Here's how the part is built. I have some questions about the finished solid (model axes, mm). Round coordinates to 2 decimals unless told otherwise and drop trailing zeros. Write each loop counter-clockwise with the first axis right and the second up, starting at its lowest first coordinate (ties: lowest second). Pieces come first, ordered by that corner, then holes. Notation, with made-up numbers: (35, -32.5) -> (90, -32.5) arc R13 ccw to (90, -28.5) -> close; hole circle Ø3 at (-1, 60.5). An arc over 180 degrees is marked (long way). Answer in a Markdown table with one row per item.
Autodesk Inventor part; units mm, degrees
ref_plane "YZ Plane" through (0, 0, 0) normal (1, 0, 0) x (0, 1, 0)
ref_plane "XZ Plane" through (0, 0, 0) normal (0, 1, 0) x (-1, 0, 0)
ref_plane "XY Plane" through (0, 0, 0) normal (0, 0, 1) x (1, 0, 0)
sketch "スケッチ1" plane through (0, 0, 0) normal (0, 0, 1) x (1, 0, 0)
  line L0 (-145, 50) -> (145, 50)
  line L1 (145, 50) -> (145, -50)
  line L2 (145, -50) -> (-145, -50)
  line L3 (-145, -50) -> (-145, 50)
  line L4 (0, -70) -> (0, 70)
  line L5 (-203, 0) -> (203, 0)
  circle A0 centre (-104.5, 10.5) radius 2.6
  circle A1 centre (-125, 21) radius 5.1
  circle A2 centre (-74.5, 10.5) radius 2.6
  circle A3 centre (-44.5, 10.5) radius 2.6
  circle A4 centre (-14.5, 10.5) radius 2.6
  circle A5 centre (15.5, 10.5) radius 2.6
  circle A6 centre (45.5, 10.5) radius 2.6
  circle A7 centre (75.5, 10.5) radius 2.6
  circle A8 centre (105.5, 10.5) radius 2.6
  line L6 (-25.25, 33.5) -> (25.25, 33.5)
  line L7 (25.25, 33.5) -> (25.25, 30)
  line L8 (25.25, 30) -> (-25.25, 30)
  line L9 (-25.25, 30) -> (-25.25, 33.5)
  circle A9 centre (125, 21) radius 5.1
  point P0 (0, 0)
  dimension "d0" = 100
  dimension "d1" = 290
  dimension "d4" = 5.2
  dimension "d5" = 60.5
  dimension "d6" = 40.5
  dimension "d21" = 10.2
  dimension "d22" = 71
  dimension "d23" = 20
  dimension "d26" = 30
  dimension "d31" = 16.5
  dimension "d32" = 50.5
  dimension "d33" = 3.5
extrude "押し出し1" add sketch "スケッチ1" along normal mid plane 3 contours L0 L4 L6 L9 L8 L5 L3 | L0 L1 L5 L4 L8 L7 L6 | L5 L4 L2 L3 | L5 L1 L2 L4
properties part number "wall_ver.1"
1) We'd pull the mould along Y, two halves only. Please class faces 1 (the face through (-103.3, 12.807, -0.021)), 2 (the face through (-2, 1, 1.5)): +Y half, -Y half, draft (parallel to the pull), parting line (faces both ways), or undercut.
Response:
| item | result |
|---|---|
| face 1 | undercut |
| face 2 | draft |
2) I want a section at C-C, the plane x = 4. List the corners of the cut face in (y, z) for me.
Response:
| item | result |
|---|---|
| outline | (-50, -1.5) -> (30, -1.5) -> (30, 1.5) -> (-50, 1.5) -> close; (33.5, -1.5) -> (50, -1.5) -> (50, 1.5) -> (33.5, 1.5) -> close |
3) I need wall thicknesses on line 1 (Y direction, x = -14.5, z = 0.1); line 2 (Y direction, x = 125, z = -0.25); line 3 (Y direction, x = -74.5, z = 0.1). Which ranges of each line are inside material? Lowest first, please. Write a range as [from, to].
Response:
| item | result |
|---|---|
| line 1 | y = [-50, 7.9], [13.1, 30], [33.5, 50] |
| line 2 | y = [-50, 15.9], [26.1, 50] |
| line 3 | y = [-50, 7.9], [13.1, 50] |
4) I want a section at A-A, the plane x = 125. List the corners of the cut face in (y, z) for me, and give its area (3 significant figures).
Response:
| item | result |
|---|---|
| outline | (-50, -1.5) -> (15.9, -1.5) -> (15.9, 1.5) -> (-50, 1.5) -> close; (26.1, -1.5) -> (50, -1.5) -> (50, 1.5) -> (26.1, 1.5) -> close |
| area | 269 mm^2 |
5) For pin 1 (6 mm diameter, centred on x = 125, y = 21, fed in from -Z), with a flat end and sliding along its axis, tell me the tip position at first contact or that it passes through.
Response:
| item | result |
|---|---|
| pin 1 | passes through |
6) I want a section at B-B, the plane z = 0.3. Count the separate pieces of the cut face and the enclosed holes in it, and give its area (3 significant figures).
Response:
| item | result |
|---|---|
| separate pieces | 1 |
| enclosed holes | 11 |
| area | 28,500 mm^2 |
